```python
from build123d import *

# Parameters (mm, degrees)
BASE_EXTRUDE_DEPTH = 12.7


with BuildPart() as part:
    # Sketch1 → Base-Extrude (new, symmetric)
    with BuildSketch(Plane.XY):
        with BuildLine():
            Line((17.6403, 16.339286512), (19.729882578, 19.063533504))
            ThreePointArc((19.729882578, 19.063533504), (19.156045845, 20.609744632), (17.6403, 21.2598))
            Line((17.6403, 21.2598), (14.70327367, 21.2598))
            ThreePointArc((14.70327367, 21.2598), (13.223883481, 20.647016519), (12.6111, 19.16762633))
            Line((12.6111, 19.16762633), (12.6111, 15.61465))
            Line((12.6111, 15.61465), (11.1125, 15.61465))
            Line((11.1125, 15.61465), (11.1125, 19.16762633))
            ThreePointArc((11.1125, 19.16762633), (12.164213258, 21.706686742), (14.70327367, 22.7584))
            Line((14.70327367, 22.7584), (17.6403, 22.7584))
            ThreePointArc((17.6403, 22.7584), (20.415434554, 21.446284653), (21.162428673, 18.4688666))
            Line((21.162428673, 18.4688666), (19.1389, 15.830735923))
            Line((19.1389, 15.830735923), (19.1389, 10.749129415))
            Line((19.1389, 10.749129415), (20.6375, 9.0662125))
            Line((20.6375, 9.0662125), (20.6375, -4.8244125))
            Line((20.6375, -4.8244125), (19.1389, -6.507329415))
            Line((19.1389, -6.507329415), (19.1389, -13.358784555))
            Line((19.1389, -13.358784555), (20.553458003, -14.773342558))
            ThreePointArc((20.553458003, -14.773342558), (18.729942105, -18.270236732), (15.019825564, -16.932883251))
            ThreePointArc((15.019825564, -16.932883251), (13.000752562, -16.523120627), (12.480559153, -18.5166))
            Line((12.480559153, -18.5166), (-12.480559153, -18.5166))
            ThreePointArc((-12.480559153, -18.5166), (-13.000752562, -16.523120627), (-15.019825564, -16.932883251))
            ThreePointArc((-15.019825564, -16.932883251), (-18.729942105, -18.270236732), (-20.553458003, -14.773342558))
            Line((-20.553458003, -14.773342558), (-19.1389, -13.358784555))
            Line((-19.1389, -13.358784555), (-19.1389, -6.507329415))
            Line((-19.1389, -6.507329415), (-20.6375, -4.8244125))
            Line((-20.6375, -4.8244125), (-20.6375, 9.0662125))
            Line((-20.6375, 9.0662125), (-19.1389, 10.749129415))
            Line((-19.1389, 10.749129415), (-19.1389, 15.830735923))
            Line((-19.1389, 15.830735923), (-21.162428673, 18.4688666))
            ThreePointArc((-21.162428673, 18.4688666), (-20.415434554, 21.446284653), (-17.6403, 22.7584))
            Line((-17.6403, 22.7584), (-14.70327367, 22.7584))
            ThreePointArc((-14.70327367, 22.7584), (-12.164213258, 21.706686742), (-11.1125, 19.16762633))
            Line((-11.1125, 19.16762633), (-11.1125, 15.61465))
            Line((-11.1125, 15.61465), (-12.6111, 15.61465))
            Line((-12.6111, 15.61465), (-12.6111, 19.16762633))
            ThreePointArc((-12.6111, 19.16762633), (-13.223883481, 20.647016519), (-14.70327367, 21.2598))
            Line((-14.70327367, 21.2598), (-17.6403, 21.2598))
            ThreePointArc((-17.6403, 21.2598), (-19.156045845, 20.609744632), (-19.729882578, 19.063533504))
            Line((-19.729882578, 19.063533504), (-17.6403, 16.339286512))
            Line((-17.6403, 16.339286512), (-17.6403, 10.17860201))
            Line((-17.6403, 10.17860201), (-19.1389, 8.495685095))
            Line((-19.1389, 8.495685095), (-19.1389, -4.253885095))
            Line((-19.1389, -4.253885095), (-17.6403, -5.93680201))
            Line((-17.6403, -5.93680201), (-17.6403, -13.979525))
            Line((-17.6403, -13.979525), (-19.1389, -15.478125))
            ThreePointArc((-19.1389, -15.478125), (-18.092238669, -16.906954381), (-16.414285827, -16.33992034))
            ThreePointArc((-16.414285827, -16.33992034), (-13.428073412, -14.819877156), (-10.898992189, -17.018))
            Line((-10.898992189, -17.018), (10.898992189, -17.018))
            ThreePointArc((10.898992189, -17.018), (13.323359075, -14.834630878), (16.30518861, -16.15877141))
            ThreePointArc((16.30518861, -16.15877141), (17.990302879, -16.935279743), (19.1389, -15.478125))
            Line((19.1389, -15.478125), (17.6403, -13.979525))
            Line((17.6403, -13.979525), (17.6403, -5.93680201))
            Line((17.6403, -5.93680201), (19.1389, -4.253885095))
            Line((19.1389, -4.253885095), (19.1389, 8.495685095))
            Line((19.1389, 8.495685095), (17.6403, 10.17860201))
            Line((17.6403, 10.17860201), (17.6403, 16.339286512))
        make_face()
    extrude(amount=BASE_EXTRUDE_DEPTH, both=True)


solid = part.part
```
Verification items for the finished model (mm, model axes). A direction names the side the tool comes from. Coordinates: 2 decimals unless noted, no trailing zeros. Loops run counter-clockwise (first coordinate to the right, second up) from the corner with the lowest first, then second, coordinate; pieces in that order, holes last. Notation, with made-up numbers: (25, 14.25) -> (36, 14.25) arc R29 ccw to (36, 53.25) -> close; hole circle Ø11 at (-29.75, -28). An arc over 180 degrees is marked (long way). Answer in a Markdown table with one row per item. Add a question column.
1. Section check C-C, the plane y = 3.5. Enter the section's corners in (x, z), then the cut area to 3 significant figures.
2. Material ranges on probe 1 along X at (y, z) = (6.5, -2.5); probe 2 along X at (y, z) = (13.5, -6.5); probe 3 along Y at (x, z) = (-18, 5.25), recorded low to high. Write a range as [from, to].
3. Section check A-A, the plane y = 17. Enter the section's corners in (x, z), then the cut area to 3 significant figures.
4. Access from +Z, -Z, +X, -X, +Y, -Y to the whole of each face (thin tool, end or side, straight path). Record for faces 1 (the face through (-12.19, 21.73, 0.18)), 2 (the face through (12, 15.615, 0)), 3 (the face through (-19.86, -14.08, 0.18)).
5. Draft check along X on faces 4 (the face through (0, -18, 12.7)), 5 (the face through (19.878, 9.919, 0.178)), 6 (the face through (-20.136, 17.131, 0.178)), 7 (the face through (-18.4, -5.084, 0.178)). Enter one of: +X half, -X half, draft (parallel to the pull), parting line (faces both ways), or undercut.
6. Section check D-D, the plane x = 0. Enter the section's corners in (y, z).
7. Section check B-B, the plane x = -14. Enter the section's corners in (y, z).
8. Depth check by flat-ended pin: P1, Ø5, axis at y = 12, z = 1.5, coming from the -X side; P2, Ø3.5, axis at y = -10, z = 4.5, coming from the +X side; P3, Ø5, axis at y = 13, z = -4, coming from the +X side; P4, Ø5, axis at x = 15, y = 13, coming from the -Z side. Enter the tip coordinate at first touch or a pass-through.
Derived:
| question | item | result |
|---|---|---|
| 1 | outline | (-20.64, -12.7) -> (-19.14, -12.7) -> (-19.14, 12.7) -> (-20.64, 12.7) -> close; (19.14, -12.7) -> (20.64, -12.7) -> (20.64, 12.7) -> (19.14, 12.7) -> close |
| 1 | area | 76.1 mm² |
| 2 | probe 1 | x = [-20.64, -19.14], [19.14, 20.64] |
| 2 | probe 2 | x = [-19.14, -17.64], [17.64, 19.14] |
| 2 | probe 3 | y = [-18.45, -16.93], [-14.34, -5.53], [9.77, 16.81], [21.23, 22.74] |
| 3 | outline | (-20.04, -12.7) -> (-18.15, -12.7) -> (-18.15, 12.7) -> (-20.04, 12.7) -> close; (-12.61, -12.7) -> (-11.11, -12.7) -> (-11.11, 12.7) -> (-12.61, 12.7) -> close; (11.11, -12.7) -> (12.61, -12.7) -> (12.61, 12.7) -> (11.11, 12.7) -> close; (18.15, -12.7) -> (20.04, -12.7) -> (20.04, 12.7) -> (18.15, 12.7) -> close |
| 3 | area | 172 mm² |
| 4 | face 1 | +Z, -Z, +Y |
| 4 | face 2 | +Z, -Z |
| 4 | face 3 | +Z, -Z, -X |
| 5 | face 4 | draft |
| 5 | face 5 | +X half |
| 5 | face 6 | -X half |
| 5 | face 7 | undercut |
| 6 | outline | (-18.52, -12.7) -> (-17.02, -12.7) -> (-17.02, 12.7) -> (-18.52, 12.7) -> close |
| 7 | outline | (-16.31, -12.7) -> (-14.8, -12.7) -> (-14.8, 12.7) -> (-16.31, 12.7) -> close; (21.14, -12.7) -> (22.69, -12.7) -> (22.69, 12.7) -> (21.14, 12.7) -> close |
| 8 | P1 | stops at x = -20.25 |
| 8 | P2 | stops at x = 19.14 |
| 8 | P3 | stops at x = 19.36 |
| 8 | P4 | passes through |
